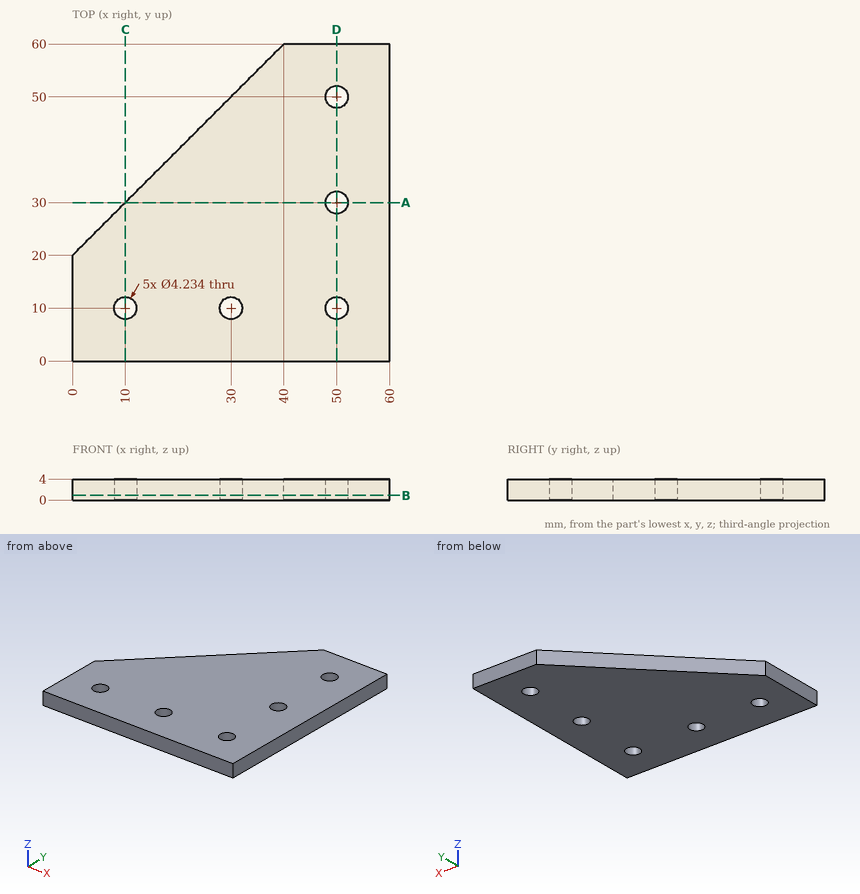
Geometry check sheet. Reference: drawing and pictorial views, mm from the part's lowest x, y, z. Give positions to 0.01 mm unless a question says otherwise; leave off trailing zeros. Write each loop counter-clockwise with the first axis right and the second up, starting at its lowest first coordinate (ties: lowest second). Pieces come first, ordered by that corner, then holes. Notation, with made-up numbers: (77.5, 57.25) - (120.5, 57.25) arc R26 cw to (120.5, 85.25) - close; hole circle Ø7 at (-19, 11). An arc over 180 degrees is marked (long way). Put each result on its own line as item: value.
Q1. Scan lines: probe 1 along Y at (x, z) = (50, 1.1); probe 2 along X at (y, z) = (50, 1). Record each from-to range of solid material in increasing order. Write a range as from..to.
Result:
probe 1: 0..7.88, 12.12..27.88, 32.12..47.88, 52.12..60
probe 2: 30..47.88, 52.12..60
Q2. Section check A-A on y = 30. Record the cut outline in (x, z).
Result:
outline: (10, 0) - (47.88, 0) - (47.88, 4) - (10, 4) - close; (52.12, 0) - (60, 0) - (60, 4) - (52.12, 4) - close
Q3. Section check C-C on x = 10. Record the cut outline in (y, z).
Result:
outline: (0, 0) - (7.88, 0) - (7.88, 4) - (0, 4) - close; (12.12, 0) - (30, 0) - (30, 4) - (12.12, 4) - close
Q4. Section check B-B on z = 0.9. Record the cut outline in (x, y), and give its area (3 significant figures).
Result:
outline: (0, 0) - (60, 0) - (60, 60) - (40, 60) - (0, 20) - close; hole circle Ø4.23 at (10, 10); hole circle Ø4.23 at (30, 10); hole circle Ø4.23 at (50, 10); hole circle Ø4.23 at (50, 30); hole circle Ø4.23 at (50, 50)
area: 2,730 mm2
Q5. Section check D-D on x = 50. Record the cut outline in (y, z), and give its area (3 significant figures).
Result:
outline: (0, 0) - (7.88, 0) - (7.88, 4) - (0, 4) - close; (12.12, 0) - (27.88, 0) - (27.88, 4) - (12.12, 4) - close; (32.12, 0) - (47.88, 0) - (47.88, 4) - (32.12, 4) - close; (52.12, 0) - (60, 0) - (60, 4) - (52.12, 4) - close
area: 189 mm2
